CAD build for the part. Positions are in the model's coordinates, mm. A direction names the side the tool comes from. Round coordinates to 2 decimals unless told otherwise and drop trailing zeros. Loops run counter-clockwise (first coordinate to the right, second up) from the corner with the lowest first, then second, coordinate; pieces in that order, holes last. Notation, with made-up numbers: M -19.75,59.5 L 11.25,59.5 A19 cw 11.25,63.5 Z; hole C -31,10.25 d4. An arc over 180 degrees is marked long. Use a Markdown table: item, result. Add a question column.
(1) Wall check: L1, parallel to Y at x = 127.5, z = 0.7; L2, parallel to X at y = 27, z = 1.75; L3, parallel to Z at x = 53, y = 67. Give the ranges that are in metal, low to high.
(2) Which spindle directions (+Z, -Z, +X, -X, +Y, -Y) get a long thin tool onto all of the face, cutting with end or side? Do faces 1 (the face through (6.53, 63.4, 1.99)), 2 (the face through (63.474, 2.981, 0.493)). Say none if no direction does.
(3) Two-plate mould, pull along Y, no slides. Class faces 3 (the face through (70, 4, 1)), 4 (the face through (123.4, 63.47, 1.99)), 5 (the face through (64.14, 68.85, 0.49)): released by +Y, released by -Y, zero draft, split by the parting line, or undercut.
(4) Band-saw the part on A-A, the plane y = 35. Write the cut outline in (x, z).
(5) Flat gauge pins, fed straight in: P1, Ø1.5, axis at x = 95, z = 2.5, coming from the -Y side; P2, Ø0.6, axis at x = 46, z = 1.5, coming from the +Y side; P3, Ø4, axis at x = 108.32, y = 2.5, coming from the +Z side. Where does each tip first touch, or does it go through?
(6) Band-saw the part on B-B, the plane x = 43.34. Write the cut outline in (y, z), and give its area (3 significant figures).
(7) Band-saw the part on D-D, the plane y = 52.5. Write the cut outline in (x, z).
(8) Band-saw the part on C-C, the plane x = 104. Write the cut outline in (y, z), and give its area (3 significant figures).
from build123d import *

# Parameters (mm, degrees)
BOSS_EXTRU_1_DEPTH      = 1
BOSS_EXTRU_2_DEPTH      = 2
ENL_V_MAT_EXTRU_1_REACH = 5
ESQUISSE3_R             = 1.6


with BuildPart() as part:
    # Esquisse1 → Boss.-Extru.1 (new body)
    with BuildSketch(Plane.XY):
        with BuildLine():
            Line((2, 0), (128, 0))
            ThreePointArc((128, 0), (129.414213562, 0.585786438), (130, 2))
            Line((130, 2), (130, 68))
            ThreePointArc((130, 68), (129.414213562, 69.414213562), (128, 70))
            Line((128, 70), (2, 70))
            ThreePointArc((2, 70), (0.585786438, 69.414213562), (0, 68))
            Line((0, 68), (0, 2))
            ThreePointArc((0, 2), (0.585786438, 0.585786438), (2, 0))
        make_face()
    extrude(amount=BOSS_EXTRU_1_DEPTH)

    # Esquisse2 → Boss.-Extru.2 (add)
    with BuildSketch(Plane.XY.offset(1)):
        with BuildLine():
            Line((10.1, 64.9), (119.9, 64.9))
            ThreePointArc((119.9, 64.9), (123.435533906, 63.435533906), (124.9, 59.9))
            Line((124.9, 59.9), (124.9, 10.1))
            ThreePointArc((124.9, 10.1), (123.435533906, 6.564466094), (119.9, 5.1))
            Line((119.9, 5.1), (10.1, 5.1))
            ThreePointArc((10.1, 5.1), (6.564466094, 6.564466094), (5.1, 10.1))
            Line((5.1, 10.1), (5.1, 59.9))
            ThreePointArc((5.1, 59.9), (6.564466094, 63.435533906), (10.1, 64.9))
        make_face()
    extrude(amount=BOSS_EXTRU_2_DEPTH)

    # Esquisse3 → Enlèv. mat.-Extru.1 (cut, up to next)
    with BuildSketch(Plane(origin=(0, 0, 0), x_dir=(-1, 0, 0), z_dir=(0, 0, -1)), mode=Mode.PRIVATE) as enl_v_mat_extru_1_sk1:
        with Locations((-65, 67.5)):
            Circle(ESQUISSE3_R)
    enl_v_mat_extru_1_tool1 = extrude(enl_v_mat_extru_1_sk1.sketch, amount=-ENL_V_MAT_EXTRU_1_REACH, mode=Mode.PRIVATE) & part.part
    add(enl_v_mat_extru_1_tool1.solids().sort_by_distance((65, 67.5, 0))[0], mode=Mode.SUBTRACT)
    # Esquisse3 → Enlèv. mat.-Extru.1 (cut, up to next)
    with BuildSketch(Plane(origin=(0, 0, 0), x_dir=(-1, 0, 0), z_dir=(0, 0, -1)), mode=Mode.PRIVATE) as enl_v_mat_extru_1_sk2:
        with Locations((-43.34, 67.5)):
            Circle(ESQUISSE3_R)
    enl_v_mat_extru_1_tool2 = extrude(enl_v_mat_extru_1_sk2.sketch, amount=-ENL_V_MAT_EXTRU_1_REACH, mode=Mode.PRIVATE) & part.part
    add(enl_v_mat_extru_1_tool2.solids().sort_by_distance((43.34, 67.5, 0))[0], mode=Mode.SUBTRACT)
    # Esquisse3 → Enlèv. mat.-Extru.1 (cut, up to next)
    with BuildSketch(Plane(origin=(0, 0, 0), x_dir=(-1, 0, 0), z_dir=(0, 0, -1)), mode=Mode.PRIVATE) as enl_v_mat_extru_1_sk3:
        with Locations((-21.68, 67.5)):
            Circle(ESQUISSE3_R)
    enl_v_mat_extru_1_tool3 = extrude(enl_v_mat_extru_1_sk3.sketch, amount=-ENL_V_MAT_EXTRU_1_REACH, mode=Mode.PRIVATE) & part.part
    add(enl_v_mat_extru_1_tool3.solids().sort_by_distance((21.68, 67.5, 0))[0], mode=Mode.SUBTRACT)
    # Esquisse3 → Enlèv. mat.-Extru.1 (cut, up to next)
    with BuildSketch(Plane(origin=(0, 0, 0), x_dir=(-1, 0, 0), z_dir=(0, 0, -1)), mode=Mode.PRIVATE) as enl_v_mat_extru_1_sk4:
        with Locations((-2.5, 67.5)):
            Circle(ESQUISSE3_R)
    enl_v_mat_extru_1_tool4 = extrude(enl_v_mat_extru_1_sk4.sketch, amount=-ENL_V_MAT_EXTRU_1_REACH, mode=Mode.PRIVATE) & part.part
    add(enl_v_mat_extru_1_tool4.solids().sort_by_distance((2.5, 67.5, 0))[0], mode=Mode.SUBTRACT)
    # Esquisse3 → Enlèv. mat.-Extru.1 (cut, up to next)
    with BuildSketch(Plane(origin=(0, 0, 0), x_dir=(-1, 0, 0), z_dir=(0, 0, -1)), mode=Mode.PRIVATE) as enl_v_mat_extru_1_sk5:
        with Locations((-2.5, 2.5)):
            Circle(ESQUISSE3_R)
    enl_v_mat_extru_1_tool5 = extrude(enl_v_mat_extru_1_sk5.sketch, amount=-ENL_V_MAT_EXTRU_1_REACH, mode=Mode.PRIVATE) & part.part
    add(enl_v_mat_extru_1_tool5.solids().sort_by_distance((2.5, 2.5, 0))[0], mode=Mode.SUBTRACT)
    # Esquisse3 → Enlèv. mat.-Extru.1 (cut, up to next)
    with BuildSketch(Plane(origin=(0, 0, 0), x_dir=(-1, 0, 0), z_dir=(0, 0, -1)), mode=Mode.PRIVATE) as enl_v_mat_extru_1_sk6:
        with Locations((-21.68, 2.5)):
            Circle(ESQUISSE3_R)
    enl_v_mat_extru_1_tool6 = extrude(enl_v_mat_extru_1_sk6.sketch, amount=-ENL_V_MAT_EXTRU_1_REACH, mode=Mode.PRIVATE) & part.part
    add(enl_v_mat_extru_1_tool6.solids().sort_by_distance((21.68, 2.5, 0))[0], mode=Mode.SUBTRACT)
    # Esquisse3 → Enlèv. mat.-Extru.1 (cut, up to next)
    with BuildSketch(Plane(origin=(0, 0, 0), x_dir=(-1, 0, 0), z_dir=(0, 0, -1)), mode=Mode.PRIVATE) as enl_v_mat_extru_1_sk7:
        with Locations((-43.34, 2.5)):
            Circle(ESQUISSE3_R)
    enl_v_mat_extru_1_tool7 = extrude(enl_v_mat_extru_1_sk7.sketch, amount=-ENL_V_MAT_EXTRU_1_REACH, mode=Mode.PRIVATE) & part.part
    add(enl_v_mat_extru_1_tool7.solids().sort_by_distance((43.34, 2.5, 0))[0], mode=Mode.SUBTRACT)
    # Esquisse3 → Enlèv. mat.-Extru.1 (cut, up to next)
    with BuildSketch(Plane(origin=(0, 0, 0), x_dir=(-1, 0, 0), z_dir=(0, 0, -1)), mode=Mode.PRIVATE) as enl_v_mat_extru_1_sk8:
        with Locations((-65, 2.5)):
            Circle(ESQUISSE3_R)
    enl_v_mat_extru_1_tool8 = extrude(enl_v_mat_extru_1_sk8.sketch, amount=-ENL_V_MAT_EXTRU_1_REACH, mode=Mode.PRIVATE) & part.part
    add(enl_v_mat_extru_1_tool8.solids().sort_by_distance((65, 2.5, 0))[0], mode=Mode.SUBTRACT)
    # Esquisse3 → Enlèv. mat.-Extru.1 (cut, up to next)
    with BuildSketch(Plane(origin=(0, 0, 0), x_dir=(-1, 0, 0), z_dir=(0, 0, -1)), mode=Mode.PRIVATE) as enl_v_mat_extru_1_sk9:
        with Locations((-86.66, 2.5)):
            Circle(ESQUISSE3_R)
    enl_v_mat_extru_1_tool9 = extrude(enl_v_mat_extru_1_sk9.sketch, amount=-ENL_V_MAT_EXTRU_1_REACH, mode=Mode.PRIVATE) & part.part
    add(enl_v_mat_extru_1_tool9.solids().sort_by_distance((86.66, 2.5, 0))[0], mode=Mode.SUBTRACT)
    # Esquisse3 → Enlèv. mat.-Extru.1 (cut, up to next)
    with BuildSketch(Plane(origin=(0, 0, 0), x_dir=(-1, 0, 0), z_dir=(0, 0, -1)), mode=Mode.PRIVATE) as enl_v_mat_extru_1_sk10:
        with Locations((-108.32, 2.5)):
            Circle(ESQUISSE3_R)
    enl_v_mat_extru_1_tool10 = extrude(enl_v_mat_extru_1_sk10.sketch, amount=-ENL_V_MAT_EXTRU_1_REACH, mode=Mode.PRIVATE) & part.part
    add(enl_v_mat_extru_1_tool10.solids().sort_by_distance((108.32, 2.5, 0))[0], mode=Mode.SUBTRACT)
    # Esquisse3 → Enlèv. mat.-Extru.1 (cut, up to next)
    with BuildSketch(Plane(origin=(0, 0, 0), x_dir=(-1, 0, 0), z_dir=(0, 0, -1)), mode=Mode.PRIVATE) as enl_v_mat_extru_1_sk11:
        with Locations((-127.5, 2.5)):
            Circle(ESQUISSE3_R)
    enl_v_mat_extru_1_tool11 = extrude(enl_v_mat_extru_1_sk11.sketch, amount=-ENL_V_MAT_EXTRU_1_REACH, mode=Mode.PRIVATE) & part.part
    add(enl_v_mat_extru_1_tool11.solids().sort_by_distance((127.5, 2.5, 0))[0], mode=Mode.SUBTRACT)
    # Esquisse3 → Enlèv. mat.-Extru.1 (cut, up to next)
    with BuildSketch(Plane(origin=(0, 0, 0), x_dir=(-1, 0, 0), z_dir=(0, 0, -1)), mode=Mode.PRIVATE) as enl_v_mat_extru_1_sk12:
        with Locations((-127.5, 67.5)):
            Circle(ESQUISSE3_R)
    enl_v_mat_extru_1_tool12 = extrude(enl_v_mat_extru_1_sk12.sketch, amount=-ENL_V_MAT_EXTRU_1_REACH, mode=Mode.PRIVATE) & part.part
    add(enl_v_mat_extru_1_tool12.solids().sort_by_distance((127.5, 67.5, 0))[0], mode=Mode.SUBTRACT)
    # Esquisse3 → Enlèv. mat.-Extru.1 (cut, up to next)
    with BuildSketch(Plane(origin=(0, 0, 0), x_dir=(-1, 0, 0), z_dir=(0, 0, -1)), mode=Mode.PRIVATE) as enl_v_mat_extru_1_sk13:
        with Locations((-108.32, 67.5)):
            Circle(ESQUISSE3_R)
    enl_v_mat_extru_1_tool13 = extrude(enl_v_mat_extru_1_sk13.sketch, amount=-ENL_V_MAT_EXTRU_1_REACH, mode=Mode.PRIVATE) & part.part
    add(enl_v_mat_extru_1_tool13.solids().sort_by_distance((108.32, 67.5, 0))[0], mode=Mode.SUBTRACT)
    # Esquisse3 → Enlèv. mat.-Extru.1 (cut, up to next)
    with BuildSketch(Plane(origin=(0, 0, 0), x_dir=(-1, 0, 0), z_dir=(0, 0, -1)), mode=Mode.PRIVATE) as enl_v_mat_extru_1_sk14:
        with Locations((-86.66, 67.5)):
            Circle(ESQUISSE3_R)
    enl_v_mat_extru_1_tool14 = extrude(enl_v_mat_extru_1_sk14.sketch, amount=-ENL_V_MAT_EXTRU_1_REACH, mode=Mode.PRIVATE) & part.part
    add(enl_v_mat_extru_1_tool14.solids().sort_by_distance((86.66, 67.5, 0))[0], mode=Mode.SUBTRACT)
    # Esquisse3 → Enlèv. mat.-Extru.1 (cut, up to next)
    with BuildSketch(Plane(origin=(0, 0, 0), x_dir=(-1, 0, 0), z_dir=(0, 0, -1)), mode=Mode.PRIVATE) as enl_v_mat_extru_1_sk15:
        with Locations((-2.5, 35)):
            Circle(ESQUISSE3_R)
    enl_v_mat_extru_1_tool15 = extrude(enl_v_mat_extru_1_sk15.sketch, amount=-ENL_V_MAT_EXTRU_1_REACH, mode=Mode.PRIVATE) & part.part
    add(enl_v_mat_extru_1_tool15.solids().sort_by_distance((2.5, 35, 0))[0], mode=Mode.SUBTRACT)
    # Esquisse3 → Enlèv. mat.-Extru.1 (cut, up to next)
    with BuildSketch(Plane(origin=(0, 0, 0), x_dir=(-1, 0, 0), z_dir=(0, 0, -1)), mode=Mode.PRIVATE) as enl_v_mat_extru_1_sk16:
        with Locations((-127.5, 35)):
            Circle(ESQUISSE3_R)
    enl_v_mat_extru_1_tool16 = extrude(enl_v_mat_extru_1_sk16.sketch, amount=-ENL_V_MAT_EXTRU_1_REACH, mode=Mode.PRIVATE) & part.part
    add(enl_v_mat_extru_1_tool16.solids().sort_by_distance((127.5, 35, 0))[0], mode=Mode.SUBTRACT)


solid = part.part
Return value:
| question | item | result |
|---|---|---|
| 1 | L1 | 0 to 0.9, 4.1 to 33.4, 36.6 to 65.9, 69.1 to 70 |
| 1 | L2 | 5.1 to 124.9 |
| 1 | L3 | 0 to 1 |
| 2 | face 1 | +Z, -X, +Y |
| 2 | face 2 | +Z, -Z |
| 3 | face 3 | zero draft |
| 3 | face 4 | released by +Y |
| 3 | face 5 | undercut |
| 4 | outline | M 0,0 L 0.9,0 L 0.9,1 L 0,1 Z; M 4.1,0 L 125.9,0 L 125.9,1 L 124.9,1 L 124.9,3 L 5.1,3 L 5.1,1 L 4.1,1 Z; M 129.1,0 L 130,0 L 130,1 L 129.1,1 Z |
| 5 | P1 | y = 5.1 |
| 5 | P2 | y = 64.9 |
| 5 | P3 | z = 1 |
| 6 | outline | M 0,0 L 0.9,0 L 0.9,1 L 0,1 Z; M 4.1,0 L 65.9,0 L 65.9,1 L 64.9,1 L 64.9,3 L 5.1,3 L 5.1,1 L 4.1,1 Z; M 69.1,0 L 70,0 L 70,1 L 69.1,1 Z |
| 6 | area | 183 mm^2 |
| 7 | outline | M 0,0 L 130,0 L 130,1 L 124.9,1 L 124.9,3 L 5.1,3 L 5.1,1 L 0,1 Z |
| 8 | outline | M 0,0 L 70,0 L 70,1 L 64.9,1 L 64.9,3 L 5.1,3 L 5.1,1 L 0,1 Z |
| 8 | area | 190 mm^2 |
